The listing builds one solid part. Answer for the finished solid, in the listing's coordinates (mm). Face numbers are marked on the shaded views. A direction names the side the tool comes from. Round coordinates to 2 decimals unless told otherwise and drop trailing zeros. Loops run counter-clockwise (first coordinate to the right, second up) from the corner with the lowest first, then second, coordinate; pieces in that order, holes last. Notation, with made-up numbers: (31, 53.25) - (82, 53.25) arc R26 ccw to (82, 72.25) - close; hole circle Ø8 at (-35, -31). An arc over 180 degrees is marked (long way). One line per question, with ' | ' between items. Start each with the question number.
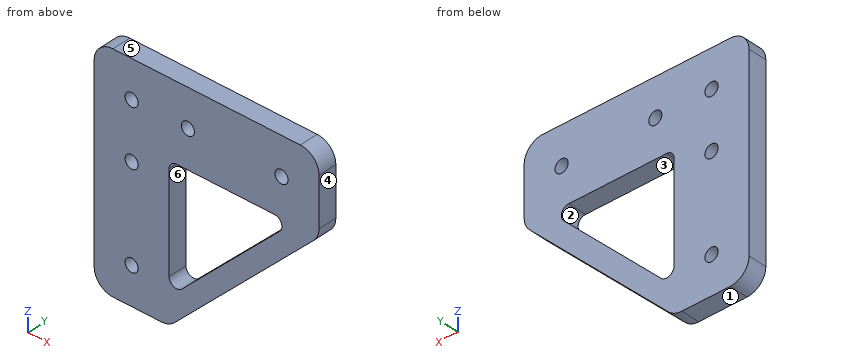
from build123d import *

# Parameters (mm, degrees)
ESBO_O1_R                = 1.75
RESSALTO_EXTRUS_O1_DEPTH = 5
FILETE2_R                = 2
ESBO_O4_R                = 1.75
CORTE_EXTRUS_O1_DEPTH    = 10
FILETE3_R                = 5


with BuildPart() as part:
    # Esboço1 → Ressalto-extrusão1 (new body)
    # profile 1 of 2: a face of its own
    with BuildSketch(Plane(origin=(0, 0, 0), x_dir=(1, 0, 0), z_dir=(0, 1, 0))):
        Polygon((52.928932188, 20), (60, 20), (60, 0), (0, 0), (0, 60), (20, 60), (20, 52.928932188), (20, 20), align=None)
        with Locations(Location((10, 10, 0), (0, 0, 270))):
            Circle(ESBO_O1_R, mode=Mode.SUBTRACT)
        with Locations(Location((50, 10, 0), (0, 0, 270))):
            Circle(ESBO_O1_R, mode=Mode.SUBTRACT)
        with Locations(Location((10, 50, 0), (0, 0, 270))):
            Circle(ESBO_O1_R, mode=Mode.SUBTRACT)
    # profile 2 of 2: a face of its own
    with BuildSketch(Plane(origin=(0, 0, 0), x_dir=(1, 0, 0), z_dir=(0, 1, 0))):
        Polygon((52.928932188, 20), (20, 52.928932188), (20, 60), (60, 20), align=None)
    extrude(amount=RESSALTO_EXTRUS_O1_DEPTH)

    # Filete2
    filete2_edges = [part.edges().sort_by_distance(p)[0] for p in [
        (52.928932188, 2.5, -20),
        (20, 2.5, -52.928932188),
        (20, 2.5, -20),
    ]]
    fillet(filete2_edges, radius=FILETE2_R)

    # Esboço4 → Corte-extrusão1 (cut)
    with BuildSketch(Plane.XZ):
        with Locations(Location((10, -25, 0), (0, 0, 270))):
            Circle(ESBO_O4_R)
        with Locations(Location((25, -10, 0), (0, 0, 270))):
            Circle(ESBO_O4_R)
    extrude(amount=-CORTE_EXTRUS_O1_DEPTH, mode=Mode.SUBTRACT)

    # Filete3
    filete3_edges = [part.edges().sort_by_distance(p)[0] for p in [
        (60, 2.5, 0),
        (0, 2.5, 0),
        (0, 2.5, -60),
        (20, 2.5, -60),
        (60, 2.5, -20),
    ]]
    fillet(filete3_edges, radius=FILETE3_R)


solid = part.part
(1) Consider L1, parallel to X at y = 4.55, z = -10; L2, parallel to Z at x = 24, y = 4.2; L3, parallel to X at y = 1.95, z = -25. Determine where each line is inside the solid, lowest interval first.
(2) Find section B-B on z = -10. Write down the section's boundary in (x, y), plus the area to 4 significant figures.
(3) Find section A-A on x = 10. Write down the section's boundary in (y, z).
(4) Find section D-D on x = 25. Write down the section's boundary in (y, z).
(5) Find section C-C on y = 2.95. Write down the section's boundary in (x, z), plus the area to 3 significant figures.
(6) Each of these flat-tipped pins is pushed along its axis until it touches: P1, Ø5.5, axis at x = 10, z = -50, coming from the -Y side; P2, Ø3, axis at y = 1, z = -24, coming from the +X side; P3, Ø1.5, axis at x = 35, y = 4.5, coming from the -Z side. Where does it stop, or does it pass through?
(7) A tool of negligible diameter and unlimited length cuts with its end or side. For the marked faces 1 and 2, from which of +Z, -Z, +X, -X, +Y, -Y can it reach the whole face along a straight path? Write none if from no direction.
(8) Determine the mould class of the marked faces 3, 4, 5 and 6 for opening direction X: pulls with the +X half, pulls with the -X half, needs draft (parallel to the pull), parting line crosses it, or undercut.
Answer below:
1) L1: 0 to 8.25, 11.75 to 23.25, 26.75 to 48.25, 51.75 to 60 | L2: -56 to -48.93, -20 to -11.44, -8.56 to 0 | L3: 0 to 8.25, 11.75 to 20, 47.93 to 55
2) outline: (0, 0) - (8.25, 0) - (8.25, 5) - (0, 5) - close; (11.75, 0) - (23.25, 0) - (23.25, 5) - (11.75, 5) - close; (26.75, 0) - (48.25, 0) - (48.25, 5) - (26.75, 5) - close; (51.75, 0) - (60, 0) - (60, 5) - (51.75, 5) - close | area: 247.5 mm2
3) outline: (0, -60) - (5, -60) - (5, -51.75) - (0, -51.75) - close; (0, -48.25) - (5, -48.25) - (5, -26.75) - (0, -26.75) - close; (0, -23.25) - (5, -23.25) - (5, -11.75) - (0, -11.75) - close; (0, -8.25) - (5, -8.25) - (5, 0) - (0, 0) - close
4) outline: (0, -55) - (5, -55) - (5, -47.93) - (0, -47.93) - close; (0, -20) - (5, -20) - (5, -11.75) - (0, -11.75) - close; (0, -8.25) - (5, -8.25) - (5, 0) - (0, 0) - close
5) outline: (0, -55) arc R5 ccw to (5, -60) - (17.93, -60) arc R5 ccw to (21.46, -58.54) - (58.54, -21.46) arc R5 ccw to (60, -17.93) - (60, -5) arc R5 ccw to (55, 0) - (5, 0) arc R5 ccw to (0, -5) - close; hole circle Ø3.5 at (10, -50); hole circle Ø3.5 at (10, -25); hole circle Ø3.5 at (10, -10); hole (20, -48.1) arc R2 ccw to (23.41, -49.51) - (49.51, -23.41) arc R2 ccw to (48.1, -20) - (22, -20) arc R2 ccw to (20, -22) - close; hole circle Ø3.5 at (25, -10); hole circle Ø3.5 at (50, -10) | area: 2,200 mm2
6) P1: y = 0 | P2: x = 57.5 | P3: z = -45.75
7) face 1: -Z, +X, -X, +Y, -Y | face 2: +Y, -Y
8) face 3: undercut | face 4: pulls with the +X half | face 5: needs draft | face 6: undercut
